Here's the drawing with two shaded views (mm, measured from the low corner). I have some questions. Give positions to 0.01 mm unless a question says otherwise; leave off trailing zeros. Loops run counter-clockwise (first coordinate to the right, second up) from the corner with the lowest first, then second, coordinate; pieces in that order, holes last. Notation, with made-up numbers: (-19.5, 17) - (23.5, 17) arc R25 ccw to (23.5, 45) - close; hole circle Ø5 at (7.25, 43.25). An arc over 180 degrees is marked (long way). Answer as a JSON object with one key per item and string values. Group by question number.
Item 1: Thinking about a two-plate mould opening in X: for the marked faces 1, 2, 3 and 4, which applies, pulls with the +X half, pulls with the -X half, needs draft (parallel to the pull), parting line crosses it, or undercut?
Item 2: Will this pin go through, and if not, where does the flat tip stop? pin 1 (8 mm diameter, centred on x = 21.5, y = 22.5, fed in from +Z).
Item 3: Please list where these lines run through material, in increasing order: L1, parallel to Y at x = 20.5, z = 17.25; L2, parallel to X at y = 18, z = 15.5; L3, parallel to Y at x = 18, z = 18.75 (1 decimal).
Item 4: Suppose I cut it at A-A on x = 21.5. Write out the boundary of the cut face in (y, z).
Item 5: Suppose I cut it at B-B on z = 17. Write out the boundary of the cut face in (x, y) (1 decimal).
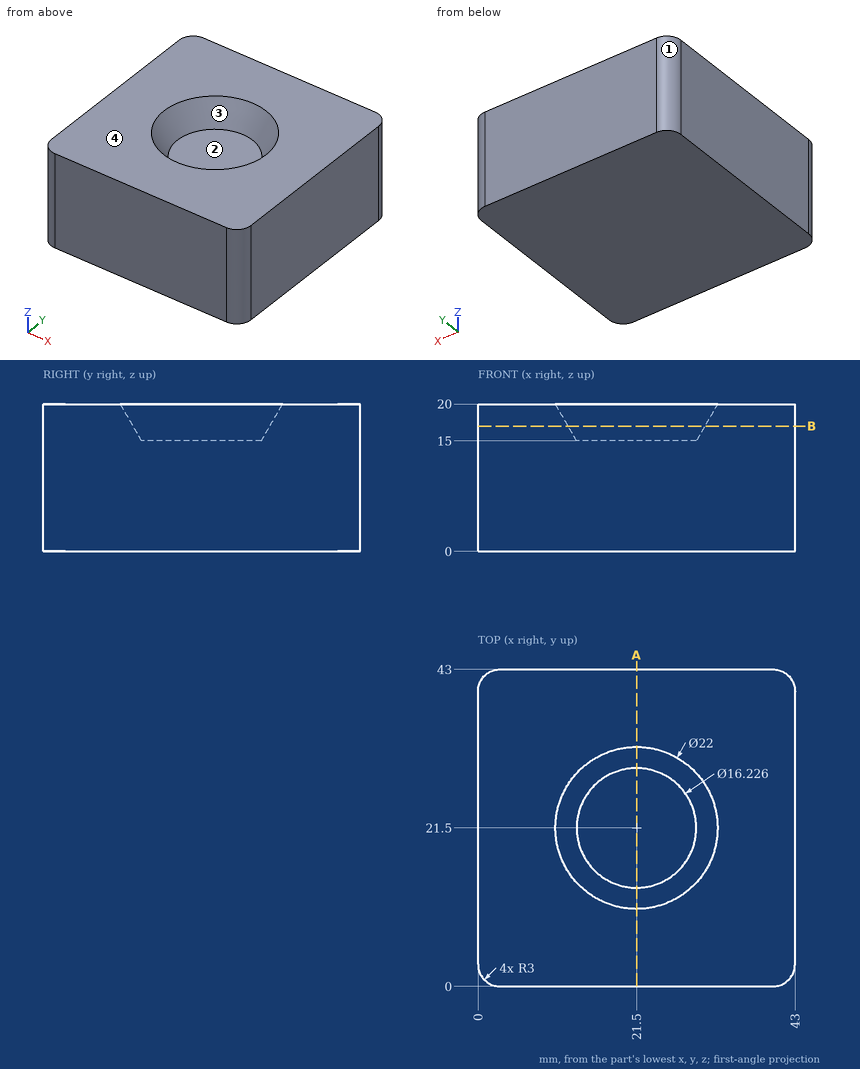
Worked out:
{
 "1": {"face 1": "pulls with the -X half", "face 2": "undercut", "face 3": "undercut", "face 4": "needs draft"},
 "2": {"pin 1": "stops at z = 15"},
 "3": {"L1": "y = 0 to 12.14, 30.86 to 43", "L2": "x = 0 to 13.86, 29.14 to 43", "L3": "y = 0 to 11.8, 31.2 to 43"},
 "4": {"outline": "(0, 0) - (43, 0) - (43, 20) - (32.5, 20) - (29.61, 15) - (13.39, 15) - (10.5, 20) - (0, 20) - close"},
 "5": {"outline": "(0, 3) arc R3 ccw to (3, 0) - (40, 0) arc R3 ccw to (43, 3) - (43, 40) arc R3 ccw to (40, 43) - (3, 43) arc R3 ccw to (0, 40) - close; hole circle Ø18.5 at (21.5, 21.5)"}
}
